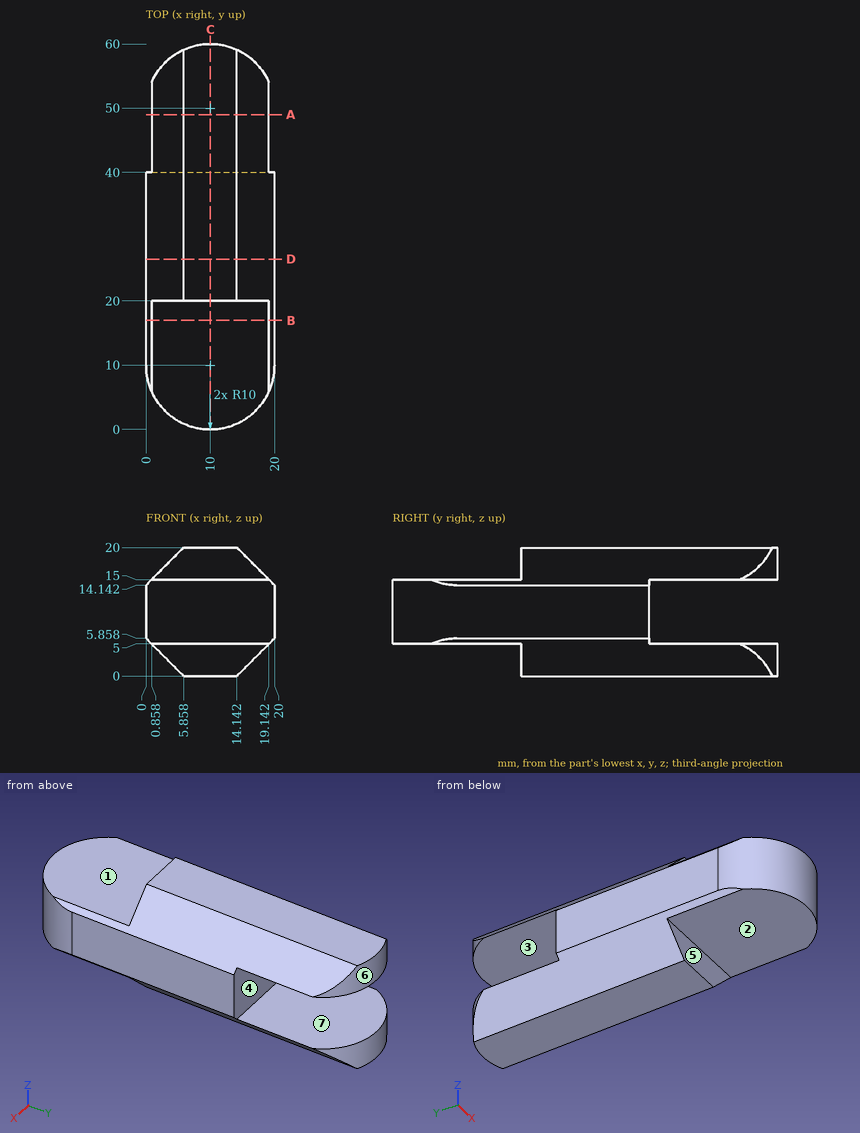
For this review, use the dimensioned drawing (mm, ordinates from the lowest corner) and the shaded views. A direction names the side the tool comes from. Coordinates: 2 decimals unless noted, no trailing zeros. Write each loop counter-clockwise with the first axis right and the second up, starting at its lowest first coordinate (ties: lowest second). Pieces come first, ordered by that corner, then holes. Notation, with made-up numbers: (-33.75, 25.5) -> (10.25, 25.5) arc R34 ccw to (10.25, 56.5) -> close; hole circle Ø5 at (16.5, 69). An arc over 180 degrees is marked (long way). Put each result on its own line as item: value.
Q1. The part is to be moulded in two halves that separate along Z. For the marked faces 1, 2, 3 and 4, say which applies: +Z half, -Z half, draft (parallel to the pull), parting line (faces both ways), or undercut.
From the geometry:
face 1: +Z half
face 2: -Z half
face 3: undercut
face 4: undercut
Q2. Clearance check with flat-ended pins moving along their axes: pin 1 Ø1.5 at (x, z) = (11.5, 3.5) entering from -Y; pin 2 Ø1.5 at (x, z) = (3, 13) entering from -Y; pin 3 Ø9 at (x, y) = (10, 7.5) entering from -Z; pin 4 Ø5.5 at (x, y) = (5.5, 50.5) entering from -Z. State where each tip first meets the part, or that it passes through.
From the geometry:
pin 1: stops at y = 20
pin 2: stops at y = 2.19
pin 3: stops at z = 5
pin 4: stops at z = 0
Q3. Take a section at D-D, the plane y = 26.5. State the section outline as (x, z) points.
From the geometry:
outline: (0, 5.86) -> (5.86, 0) -> (14.14, 0) -> (20, 5.86) -> (20, 14.14) -> (14.14, 20) -> (5.86, 20) -> (0, 14.14) -> close
Q4. Wall thickness on L1, parallel to Z at x = 10.5, y = 44.5; L2, parallel to Z at x = 11, y = 19; L3, parallel to Z at x = 4.5, y = 28: over which ranges is each line inside the solid? List them lowest first.
From the geometry:
L1: z = 0 to 5, 15 to 20
L2: z = 5 to 15
L3: z = 1.36 to 18.64
Q5. Take a section at B-B, the plane y = 17. State the section outline as (x, z) points.
From the geometry:
outline: (0, 5.86) -> (0.86, 5) -> (19.14, 5) -> (20, 5.86) -> (20, 14.14) -> (19.14, 15) -> (0.86, 15) -> (0, 14.14) -> close
Q6. Take a section at A-A, the plane y = 49. State the section outline as (x, z) points, then the cut area to 3 significant figures.
From the geometry:
outline: (0.86, 5) -> (5.86, 0) -> (14.14, 0) -> (19.14, 5) -> close; (0.86, 15) -> (19.14, 15) -> (14.14, 20) -> (5.86, 20) -> close
area: 133 mm2
Q7. Take a section at C-C, the plane x = 10. State the section outline as (y, z) points, then the cut area to 3 significant figures.
From the geometry:
outline: (0, 5) -> (20, 5) -> (20, 0) -> (60, 0) -> (60, 5) -> (40, 5) -> (40, 15) -> (60, 15) -> (60, 20) -> (20, 20) -> (20, 15) -> (0, 15) -> close
area: 800 mm2
Q8. Tool access review of the marked faces 5, 6 and 7: name each direction out of +Z, -Z, +X, -X, +Y, -Y from which nothing blocks a thin tool from reaching the whole face with its end or side.
From the geometry:
face 5: -Z, +X, -X, -Y
face 6: +Z, -Z, +Y
face 7: +X, -X, +Y
